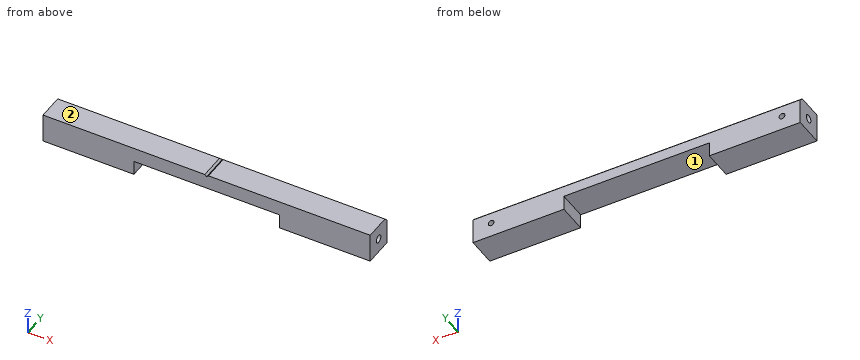
from build123d import *

# Parameters (mm, degrees)
SKETCH1_W                 = 25.4
SKETCH1_H                 = 25.4
EXTRUDE1_DEPTH            = 142.875
CHAMFER1_SIZE             = 3.175
M6X1_0_TAPPED_HOLE1_D     = 5
M6X1_0_TAPPED_HOLE1_DEPTH = 14.986
M6X1_0_TAPPED_HOLE1_TIP   = 1.502151548
CUT_EXTRUDE1_REACH        = 27.4
SKETCH10_W                = 127
SKETCH10_H                = 12.7
CUT_EXTRUDE2_REACH        = 27.4


with BuildPart() as part:
    # Sketch1 → Extrude1 (new body, symmetric)
    with BuildSketch(Plane(origin=(0, 0, 0), x_dir=(0, 0, -1), z_dir=(1, 0, 0))):
        Rectangle(SKETCH1_W, SKETCH1_H)
    extrude(amount=EXTRUDE1_DEPTH, both=True)

    # Sketch2 → M8x1.25 Tapped Hole1 (revolve, cut)
    with BuildSketch(Plane(origin=(142.875, 0, 0), x_dir=(0, 0, -1), z_dir=(0, 1, 0))):
        Polygon((0, 0), (0, 21.804126105), (3.4, 19.7612), (3.4, 0), align=None)
    m8x1_25_tapped_hole1 = revolve(axis=Axis((149.225, 0, 0), (-1, 0, 0)), mode=Mode.SUBTRACT)

    # Mirror1: M8x1.25 Tapped Hole1 across plane
    add(m8x1_25_tapped_hole1.mirror(Plane(origin=(0, 0, 0), x_dir=(0, 0, 1), z_dir=(1, 0, 0))), mode=Mode.SUBTRACT)

    # Chamfer1
    chamfer1_edges = [part.edges().sort_by_distance(p)[0] for p in [
        (0, 12.7, 12.7),
    ]]
    chamfer(chamfer1_edges, length=CHAMFER1_SIZE)

    # M6x1.0 Tapped Hole1
    with Locations(Plane(origin=(0, 12.7, 0), x_dir=(-1, 0, 0), z_dir=(0, 1, 0))):
        with Locations((127, 0), (-127, 0)):
            Hole(M6X1_0_TAPPED_HOLE1_D / 2, depth=M6X1_0_TAPPED_HOLE1_DEPTH)
            with Locations((0, 0, -(M6X1_0_TAPPED_HOLE1_DEPTH + M6X1_0_TAPPED_HOLE1_TIP / 2))):  # 118° drill point
                Cone(0, M6X1_0_TAPPED_HOLE1_D / 2, M6X1_0_TAPPED_HOLE1_TIP, mode=Mode.SUBTRACT)

    # Sketch10 → Cut-Extrude1 (cut, up to next)
    with BuildSketch(Plane(origin=(0, 12.7, 0), x_dir=(1, 0, 0), z_dir=(0, 1, 0)), mode=Mode.PRIVATE) as cut_extrude1_sk1:
        with Locations((0, 6.35)):
            Rectangle(SKETCH10_W, SKETCH10_H)
    cut_extrude1_tool1 = extrude(cut_extrude1_sk1.sketch, amount=-CUT_EXTRUDE1_REACH, mode=Mode.PRIVATE) & part.part
    add(cut_extrude1_tool1.solids().sort_by_distance((0, 12.7, -6.35))[0], mode=Mode.SUBTRACT)

    # Sketch11 → Cut-Extrude2 (cut, up to next)
    with BuildSketch(Plane.XZ.offset(12.7), mode=Mode.PRIVATE) as cut_extrude2_sk1:
        Polygon((-1.5875, 12.7), (1.5875, 12.7), (0, 11.1125), align=None)
    cut_extrude2_tool1 = extrude(cut_extrude2_sk1.sketch, amount=-CUT_EXTRUDE2_REACH, mode=Mode.PRIVATE) & part.part
    add(cut_extrude2_tool1.solids().sort_by_distance((0, -12.7, 12.170833))[0], mode=Mode.SUBTRACT)


solid = part.part
Geometry: final body of the model. Coordinates: model frame, mm. Face numbers are marked on the shaded views. Round coordinates to 2 decimals unless told otherwise and drop trailing zeros. Order: outer loops, then holes, each group sorted by start corner. A loop starts at its lowest first (then second) coordinate and runs counter-clockwise, first axis right, second up. Notation, with made-up numbers: (63.25, -5) - (76.25, -5) arc R19 cw to (76.25, 8) - close; hole circle Ø10 at (59, 53). An arc over 180 degrees is marked (long way). Write each question's results on one line, items separated by ' | '.
Item 1: Section A-A, the plane x = 16.5. Return the cut outline in (y, z) (3 decimals).
Completed:
outline: (-12.7, 0) - (12.7, 0) - (12.7, 9.525) - (9.525, 12.7) - (-12.7, 12.7) - close
Item 2: First-contact query: pin 1 Ø4 at (y, z) = (0, 0) entering from +X; pin 2 Ø2 at (x, y) = (44, -3.5) entering from -Z. Flat tips, straight axial feed; report the tip coordinate or a pass-through.
Completed:
pin 1: x = 122.27 | pin 2: z = 0
Item 3: Material intervals for line 1 along Z through (x, y) = (-135.5, 0); line 2 along Z through (x, y) = (127, 5), sorted ascending. Write a range as [from, to].
Completed:
line 1: [-12.7, -3.4], [3.4, 12.7] | line 2: [-12.7, -2.5], [2.5, 12.7]
Item 4: Mould query, pull axis X, two halves, no side actions, for the marked faces 1 and 2. Classes: pulls with the +X half, pulls with the -X half, needs draft (parallel to the pull), parting line crosses it, or undercut.
Completed:
face 1: undercut | face 2: needs draft
